Autodesk Inventor part; units mm, degrees
ref_plane "to_bearing_XY" through (0, 34, -6.5) normal (0, 0, -1) x (1, 0, 0)
ref_plane "to_bearing_YZ" through (0, 34, -6.5) normal (1, 0, 0) x (0, -1, 0)
ref_plane "to_bearing_ZX" through (0, 34, -6.5) normal (0, -1, 0) x (0, 0, -1)
sketch "Sketch_9" plane through (0, 0, 0) normal (0, 0, 1) x (1, 0, 0)
  line L0 (-19, 34) -> (-19, 0)
  line L1 (-19, 0) -> (19, 0)
  line L2 (19, 0) -> (19, 34)
  arc A0 (19, 34) -> (-19, 34) centre (0, 34) ccw
extrude "Extrusion1" add sketch "Sketch_9" against normal blind 15
sketch "Sketch_1" plane through (0, 0, 0) normal (1, 0, 0) x (0, 0, -1)
  line L0 (0, 14) -> (0, 0)
  line L1 (0, 0) -> (5, 0)
  line L2 (5, 0) -> (5, 14)
  line L3 (5, 14) -> (0, 14)
extrude "Extrusion2" cut sketch "Sketch_1" along normal mid plane 76
sketch "Sketch_2" plane through (0, 0, 0) normal (1, 0, 0) x (0, 0, -1)
  line L0 (15, 34) -> (2, 34)
  line L1 (2, 34) -> (2, 49)
  line L2 (2, 49) -> (11, 49)
  line L3 (11, 49) -> (11, 49.7)
  line L4 (11, 49.7) -> (12.35, 49.7)
  line L5 (12.35, 49.7) -> (12.35, 49)
  line L6 (12.35, 49) -> (15, 49)
  line L7 (15, 49) -> (15, 34)
  line L8 (15, 34) -> (2, 34)
revolve "Revolution1" cut sketch "Sketch_2" angle 360 about axis through (0, 34, -15) along (0, 0, -1)
sketch "Sketch4" plane through (0, 0, 0) normal (0, 0, 1) x (1, 0, 0)
  point P0 (0, 34)
hole "Hole1" at (0, 34, 0) direction (0, 0, -1) diameter 24 depth 15
sketch "Sketch5" plane through (0, 0, -15) normal (0, 0, -1) x (-1, 0, 0)
  point P0 (7, 7)
hole "Hole2" at (-7, 7, -15) direction (0, 0, 1) diameter 6 depth 15
pattern_linear "Rectangular Pattern1" count 2 spacing 14 along (1, 0, 0) of "Hole2"
ref_plane "to_bearing_XY" through (0, 34, -6.5) normal (0, 0, -1) x (1, 0, 0)
ref_plane "to_bearing_YZ" through (0, 34, -6.5) normal (1, 0, 0) x (0, -1, 0)
ref_plane "to_bearing_ZX" through (0, 34, -6.5) normal (0, -1, 0) x (0, 0, -1)
ref_plane "to_retaining_ring_XY" through (0, 34, -11) normal (0, 0, 1) x (-1, 0, 0)
ref_plane "to_retaining_ring_YZ" through (0, 34, -11) normal (-1, 0, 0) x (0, -1, 0)
ref_plane "to_retaining_ring_ZX" through (0, 34, -11) normal (0, -1, 0) x (0, 0, 1)
properties part number "SBGSNA6200ZZ-20_h"
Work out the finished part from the listing and answer in its coordinate system (mm). A direction names the side the tool comes from. Give positions to 0.01 mm unless a question says otherwise; leave off trailing zeros. Loops run counter-clockwise (first coordinate to the right, second up) from the corner with the lowest first, then second, coordinate; pieces in that order, holes last. Notation, with made-up numbers: (43, 37) - (82, 37) arc R26 ccw to (82, 61) - close; hole circle Ø1 at (33, -13). An arc over 180 degrees is marked (long way). One line per question, with ' | ' between items.
(1) Straight lines are drawn through the part: probe 1 along X at (y, z) = (7, -7.75); probe 2 along X at (y, z) = (33.5, -0.75); probe 3 along Z at (x, y) = (-7, 20.5). For each, find the intervals that lie inside material, in ascending order.
Recorded:
probe 1: x = -19 to -10, -4 to 4, 10 to 19 | probe 2: x = -19 to -11.99, 11.99 to 19 | probe 3: z = -15 to -12.35, -11 to 0
(2) A tool of negligible diameter and unlimited length cuts with its end or side. For faces 4 (the face through (10, 27, -2)), 5 (the face through (0, 7, -5)), 6 (the face through (-8, 47, -11)), from which of +Z, -Z, +X, -X, +Y, -Y can it reach the whole face along a straight path? Write none if from no direction.
Recorded:
face 4: -Z | face 5: +Z, +X, -X, -Y | face 6: none
(3) Each of these flat-tipped pins is pushed along its axis until it touches: pin 1 Ø6 at (y, z) = (44, -5) entering from +X; pin 2 Ø15.5 at (x, y) = (-9, 5.5) entering from +Z; pin 3 Ø1.5 at (x, z) = (3, -2) entering from -Y. Where does it stop, or does it pass through?
Recorded:
pin 1: stops at x = 17.66 | pin 2: stops at z = -5 | pin 3: stops at y = 14
(4) The part is cut by section C-C (y = 6). Write down the section's boundary in (x, z).
Recorded:
outline: (-19, -15) - (-9.83, -15) - (-9.83, -5) - (-19, -5) - close; (-4.17, -15) - (4.17, -15) - (4.17, -5) - (-4.17, -5) - close; (9.83, -15) - (19, -15) - (19, -5) - (9.83, -5) - close
(5) The mould has two halves that part along Y. Classify faces 1 (the face through (19, 17, -9)), 2 (the face through (0, 14, -3)), 3 (the face through (0.69, 18.315, -11.684)): +Y half, -Y half, draft (parallel to the pull), parting line (faces both ways), or undercut.
Recorded:
face 1: draft | face 2: -Y half | face 3: undercut
(6) The part is cut by section B-B (z = -9.75). Write down the section's boundary in (x, y), then the cut area to 3 significant figures.
Recorded:
outline: (-19, 0) - (19, 0) - (19, 34) arc R19 ccw to (-19, 34) - close; hole circle Ø30 at (0, 34); hole circle Ø6 at (-7, 7); hole circle Ø6 at (7, 7) | area: 1,100 mm²
(7) The part is cut by section A-A (x = 0). Write down the section's boundary in (y, z).
Recorded:
outline: (0, -15) - (19, -15) - (19, -12.35) - (18.3, -12.35) - (18.3, -11) - (19, -11) - (19, -2) - (22, -2) - (22, 0) - (14, 0) - (14, -5) - (0, -5) - close; (46, -2) - (49, -2) - (49, -11) - (49.7, -11) - (49.7, -12.35) - (49, -12.35) - (49, -15) - (53, -15) - (53, 0) - (46, 0) - close
(8) The part is cut by section D-D (x = 8). Write down the section's boundary in (y, z).
Recorded:
outline: (0, -15) - (4.17, -15) - (4.17, -5) - (0, -5) - close; (9.83, -15) - (21.31, -15) - (21.31, -12.35) - (20.49, -12.35) - (20.49, -11) - (21.31, -11) - (21.31, -2) - (25.06, -2) - (25.06, 0) - (14, 0) - (14, -5) - (9.83, -5) - close; (42.94, -2) - (46.69, -2) - (46.69, -11) - (47.51, -11) - (47.51, -12.35) - (46.69, -12.35) - (46.69, -15) - (51.23, -15) - (51.23, 0) - (42.94, 0) - close
